Autodesk Inventor part; units mm, degrees
ref_plane "YZ Plane" through (0, 0, 0) normal (1, 0, 0) x (0, 1, 0)
ref_plane "XZ Plane" through (0, 0, 0) normal (0, 1, 0) x (-1, 0, 0)
ref_plane "XY Plane" through (0, 0, 0) normal (0, 0, 1) x (1, 0, 0)
sketch "Sketch1" plane through (0, 0, 0) normal (0, 1, 0) x (-1, 0, 0)
  line L0 (0, 0) -> (15, 0)
  line L1 (15, 0) -> (15, -4)
  line L2 (15, -4) -> (0, -4)
  line L3 (0, -4) -> (0, 0)
  dimension "d0" = 15
  dimension "d1" = 4
extrude "Extrusion1" add sketch "Sketch1" along normal blind 1
sketch "Sketch2" plane through (0, 1, 0) normal (0, 1, 0) x (1, 0, 0)
  line L0 (0, 4) -> (-15, 4)
  line L1 (-15, 4) -> (-15, 0)
  point P0 (0, 0)
  point P1 (-13, 2)
  dimension "d18" = 2
  dimension "d19" = 2
hole "Hole1" at (-13, 1, -2) direction (0, -1, 0) diameter 3 depth 5 tip angle 118
sketch "Sketch3" plane through (0, 1, 0) normal (0, 1, 0) x (1, 0, 0)
  line L0 (0, 0) -> (0, 4)
  line L1 (0, 4) -> (-15, 4)
  point P0 (-3, 2)
  dimension "d20" = 3
  dimension "d21" = 2
hole "Hole2" at (-3, 1, -2) direction (0, -1, 0) diameter 3 depth 5 tip angle 118
sketch "Sketch4" plane through (0, 1, 0) normal (0, 1, 0) x (1, 0, 0)
  point P0 (0, 0)
fillet "Fillet1" radius 1 4 edges at (0, 0.5, 0) (0, 0.5, -4) (-15, 0.5, 0) (-15, 0.5, -4)
sketch "Sketch5" plane through (0, 1, 0) normal (0, 1, 0) x (1, 0, 0)
  line L0 (-11, 1) -> (-11, 3) construction
  line L1 (-11, 3) -> (-5, 3) construction
  line L2 (-5, 3) -> (-5, 1) construction
  line L3 (-5, 1) -> (-11, 1) construction
  line L4 (-1, 4) -> (-14, 4)
  line L5 (-14, 0) -> (-1, 0)
  line L6 (0, 1) -> (0, 3)
  line L7 (-15, 3) -> (-15, 1)
  spline S0 degree 2 poles (-9.9643, 1.4919) (-9.9643, 1.3947) (-10.03, 1.2301) (-10.0956, 1.1702) knots 0 0 0 1 2 2 2
  spline S1 degree 2 poles (-10.0956, 1.1702) (-10.1605, 1.1102) (-10.3549, 1.0446) (-10.4814, 1.0446) knots 0 0 0 1 2 2 2
  spline S2 degree 2 poles (-10.4814, 1.0446) (-10.607, 1.0446) (-10.7934, 1.1086) (-10.8622, 1.1694) knots 0 0 0 1 2 2 2
  spline S3 degree 2 poles (-10.8622, 1.1694) (-10.9295, 1.2293) (-11, 1.393) (-11, 1.4943) knots 0 0 0 1 2 2 2
  spline S4 degree 2 poles (-11, 1.4943) (-11, 1.5446) (-10.9854, 1.6329) (-10.9741, 1.6702) knots 0 0 0 1 2 2 2
  spline S5 degree 2 poles (-10.9741, 1.6702) (-10.9635, 1.7026) (-10.9335, 1.7699) (-10.9157, 1.8031) knots 0 0 0 1 2 2 2
  line L8 (-10.9157, 1.8031) -> (-10.7553, 1.8031)
  line L9 (-10.7553, 1.8031) -> (-10.7553, 1.7925)
  spline S6 degree 2 poles (-10.7553, 1.7925) (-10.7715, 1.7747) (-10.8169, 1.7196) (-10.8387, 1.6799) knots 0 0 0 1 2 2 2
  spline S7 degree 2 poles (-10.8387, 1.6799) (-10.8598, 1.6418) (-10.8865, 1.5519) (-10.8865, 1.4935) knots 0 0 0 1 2 2 2
  spline S8 degree 2 poles (-10.8865, 1.4935) (-10.8865, 1.4295) (-10.8339, 1.3152) (-10.7836, 1.2723) knots 0 0 0 1 2 2 2
  spline S9 degree 2 poles (-10.7836, 1.2723) (-10.7326, 1.2301) (-10.5778, 1.1831) (-10.4814, 1.1831) knots 0 0 0 1 2 2 2
  spline S10 degree 2 poles (-10.4814, 1.1831) (-10.3784, 1.1831) (-10.2301, 1.2326) (-10.1791, 1.2755) knots 0 0 0 1 2 2 2
  spline S11 degree 2 poles (-10.1791, 1.2755) (-10.1297, 1.3177) (-10.0794, 1.4303) (-10.0794, 1.4935) knots 0 0 0 1 2 2 2
  spline S12 degree 2 poles (-10.0794, 1.4935) (-10.0794, 1.5511) (-10.1078, 1.6491) (-10.1288, 1.6872) knots 0 0 0 1 2 2 2
  spline S13 degree 2 poles (-10.1288, 1.6872) (-10.1499, 1.7237) (-10.1937, 1.778) (-10.2091, 1.7934) knots 0 0 0 1 2 2 2
  line L10 (-10.2091, 1.7934) -> (-10.2091, 1.8031)
  line L11 (-10.2091, 1.8031) -> (-10.0502, 1.8031)
  spline S14 degree 2 poles (-10.0502, 1.8031) (-10.0348, 1.7699) (-10.0065, 1.7115) (-9.9935, 1.6702) knots 0 0 0 1 2 2 2
  spline S15 degree 2 poles (-9.9935, 1.6702) (-9.9789, 1.6264) (-9.9643, 1.5519) (-9.9643, 1.4919) knots 0 0 0 1 2 2 2
  line L12 (-10.359, 2.265) -> (-10.359, 1.8865)
  line L13 (-10.359, 1.8865) -> (-10.4806, 1.8865)
  line L14 (-10.4806, 1.8865) -> (-10.4806, 2.265)
  line L15 (-10.4806, 2.265) -> (-10.359, 2.265)
  line L16 (-9.9822, 2.9643) -> (-9.9822, 2.4765)
  line L17 (-9.9822, 2.4765) -> (-10.0843, 2.4765)
  line L18 (-10.0843, 2.4765) -> (-10.0843, 2.658)
  line L19 (-10.0843, 2.658) -> (-10.7545, 2.658)
  line L20 (-10.7545, 2.658) -> (-10.7545, 2.4765)
  line L21 (-10.7545, 2.4765) -> (-10.846, 2.4765)
  spline S16 degree 2 poles (-10.846, 2.4765) (-10.846, 2.5794) (-10.9044, 2.6767) (-10.9854, 2.6831) knots 0 0 0 1 2 2 2
  line L22 (-10.9854, 2.6831) -> (-10.9854, 2.7869)
  line L23 (-10.9854, 2.7869) -> (-10.0843, 2.7869)
  line L24 (-10.0843, 2.7869) -> (-10.0843, 2.9643)
  line L25 (-10.0843, 2.9643) -> (-9.9822, 2.9643)
  point P0 (0, 0)
  point P1 (-8, 1)
  dimension "d23" = 1
  dimension "d24" = 1
  dimension "d25" = 5
  dimension "d26" = 4
extrude "Extrusion2" cut sketch "Sketch5" against normal blind 0.5
properties part number "Parts_Combiner"
Input: part model. Units: mm. Frame: model coordinates. Give positions to 0.01 mm unless a question says otherwise; leave off trailing zeros. Order: outer loops, then holes, each group sorted by start corner. A loop starts at its lowest first (then second) coordinate and runs counter-clockwise, first axis right, second up. Notation, with made-up numbers: (-5, -12) - (22, -12) arc R18 ccw to (22, 18) - close; hole circle Ø11 at (45, 25.5). An arc over 180 degrees is marked (long way). Use a Markdown table: item, result.
(1) Draft query along Z for faces 1 (the flat face through (-15, 0.5, -2)), 2 (the cylindrical face through (-1.67, 0.49, -1.31)), 3 (the cylindrical face through (-12.425, 0.493, -0.614)), 4 (the flat face through (-7.6, 0.5, -4)). Return one class per face: released by +Z, released by -Z, zero draft, split by the parting line, or undercut.
Computed values:
| item | result |
|---|---|
| face 1 | zero draft |
| face 2 | undercut |
| face 3 | undercut |
| face 4 | released by -Z |
(2) Section query A-A (x = -13). Output: boundary loops of the cut face in (y, z), then the cut area to 3 significant figures.
Computed values:
| item | result |
|---|---|
| outline | (0, -4) - (1, -4) - (1, -3.5) - (0, -3.5) - close; (0, -0.5) - (1, -0.5) - (1, 0) - (0, 0) - close |
| area | 1.00 mm2 |
(3) Section query B-B (z = -0.8). Output: boundary loops of the cut face in (x, y).
Computed values:
| item | result |
|---|---|
| outline | (-14.98, 0) - (-13.9, 0) - (-13.9, 1) - (-14.98, 1) - close; (-12.1, 0) - (-3.9, 0) - (-3.9, 1) - (-12.1, 1) - close; (-2.1, 0) - (-0.02, 0) - (-0.02, 1) - (-2.1, 1) - close |
(4) Line query: line 1 (X direction, y = 0.4, z = -2); line 2 (Z direction, x = -13, y = 0.35); line 3 (X direction, y = 0.65, z = -0.8). Output: solid intervals per line, ascending. Write a range as from..to.
Computed values:
| item | result |
|---|---|
| line 1 | x = -15..-14.5, -11.5..-4.5, -1.5..0 |
| line 2 | z = -4..-3.5, -0.5..0 |
| line 3 | x = -14.98..-13.9, -12.1..-3.9, -2.1..-0.02 |
